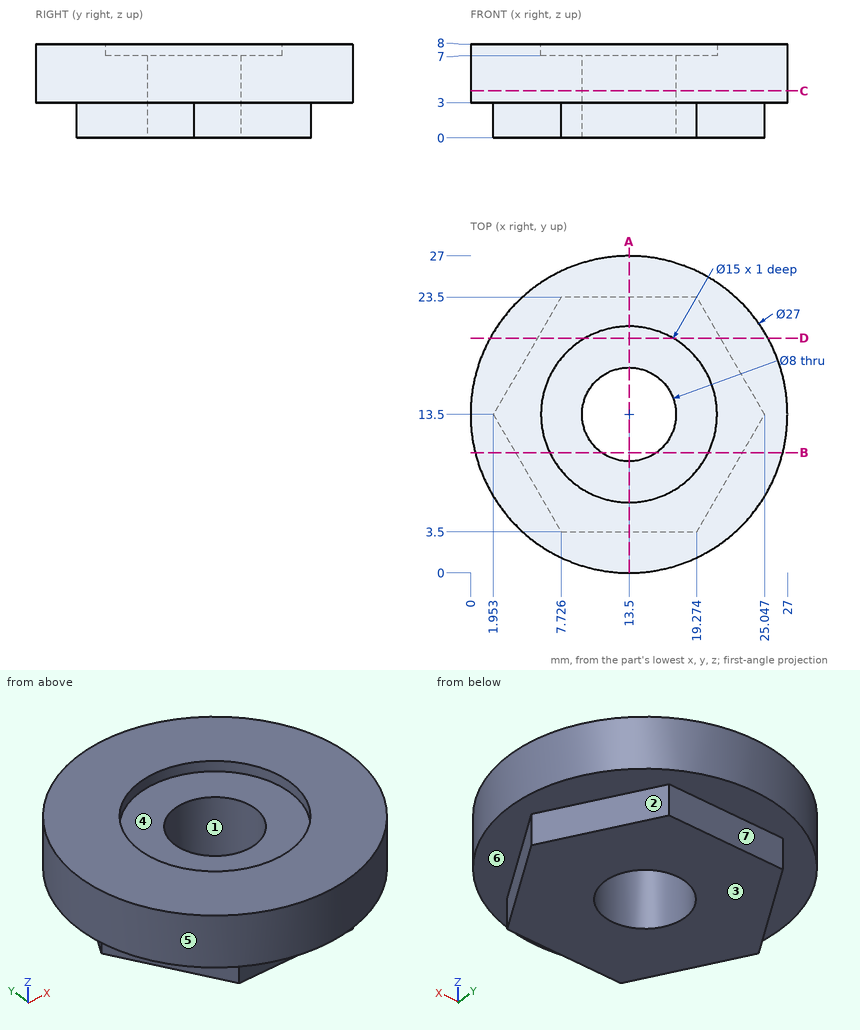
The drawing under review shows one solid part. Ordinate dimensions are in mm from its lowest x, y, z. A direction names the side the tool comes from. Coordinates: 2 decimals unless noted, no trailing zeros. Loops run counter-clockwise (first coordinate to the right, second up) from the corner with the lowest first, then second, coordinate; pieces in that order, holes last. Notation, with made-up numbers: M 23.25,-38.5 L 45.25,-38.5 A6 cw 45.25,-30.5 Z; hole C -33,-37.75 d7. An arc over 180 degrees is marked long. Use one line per item in the form item = value.
(1) For the marked faces 4, 5, 6 and 7, list the 3-axis set-ups (+Z, -Z, +X, -X, +Y, -Y) from which the entire face can be reached by the end or side of a thin tool; tool diameter is ignored.
Return value:
face_4 = +Z
face_5 = +Z, -Z
face_6 = -Z
face_7 = -Z, +X, -X, +Y
(2) Consider section D-D (y = 20). Write out the cut boundary in (x, z) (1 decimal), and give its area (3 significant figures).
Return value:
outline = M 1.7,3 L 5.7,3 L 5.7,0 L 21.3,0 L 21.3,3 L 25.3,3 L 25.3,8 L 17.2,8 L 17.2,7 L 9.8,7 L 9.8,8 L 1.7,8 Z
area = 158 mm2
(3) Consider section B-B (y = 10.25). Write out the cut boundary in (x, z), and give its area (3 significant figures).
Return value:
outline = M 0.4,3 L 3.83,3 L 3.83,0 L 11.17,0 L 11.17,7 L 6.74,7 L 6.74,8 L 0.4,8 Z; M 15.83,0 L 23.17,0 L 23.17,3 L 26.6,3 L 26.6,8 L 20.26,8 L 20.26,7 L 15.83,7 Z
area = 143 mm2
(4) For line 1 along Y through (x, z) = (13.5, 2); line 2 along Y through (x, z) = (13.5, 7.4); line 3 along Z through (x, y) = (10, 25.25), list the stretches that pass through material, from the lowest coordinate up. Write a range as from..to.
Return value:
line_1 = 3.5..9.5, 17.5..23.5
line_2 = 0..6, 21..27
line_3 = 3..8
(5) Consider section C-C (z = 4). Write out the cut boundary in (x, y), and give its area (3 significant figures).
Return value:
outline = C 13.5,13.5 d27; hole C 13.5,13.5 d8
area = 522 mm2
(6) Draft analysis for pull direction Y (two halves, no side actions). For the marked faces 1, 2 and 3, state which applies: pulls with the +Y half, pulls with the -Y half, needs draft (parallel to the pull), parting line crosses it, or undercut.
Return value:
face_1 = undercut
face_2 = pulls with the +Y half
face_3 = needs draft
(7) Clearance check with flat-ended pins moving along their axes: P1, Ø2, axis at x = 17.5, z = 2.5, coming from the +Y side; P2, Ø1.5, axis at x = 14.5, z = 5, coming from the -Y side; P3, Ø1.5, axis at x = 22.5, z = 1, coming from the +Y side. State where each tip first meets the part, or that it passes through.
Return value:
P1 = 26.63
P2 = 0
P3 = 19.21
(8) Consider section A-A (x = 13.5). Write out the cut boundary in (y, z).
Return value:
outline = M 0,3 L 3.5,3 L 3.5,0 L 9.5,0 L 9.5,7 L 6,7 L 6,8 L 0,8 Z; M 17.5,0 L 23.5,0 L 23.5,3 L 27,3 L 27,8 L 21,8 L 21,7 L 17.5,7 Z
